Can you work these out from the model? Positions are in its coordinate system, mm. Face numbers are marked on the shaded views. A direction names the side the tool comes from. Round coordinates to 2 decimals unless told otherwise and drop trailing zeros. Loops run counter-clockwise (first coordinate to the right, second up) from the corner with the lowest first, then second, coordinate; pieces in that order, holes last. Notation, with made-up numbers: (-6.5, 9.25) -> (50.5, 9.25) arc R16 cw to (50.5, 13.25) -> close; hole circle Ø9 at (44, 52). An arc over 180 degrees is marked (long way). Write item = value, one per line.
from build123d import *

# Parameters (mm, degrees)
SKETCH2_R           = 2.1
BOSS_EXTRUDE1_DEPTH = 5
SKETCH3_R           = 5
SKETCH3_R_2         = 2.1
BOSS_EXTRUDE2_DEPTH = 5


with BuildPart() as part:
    # Sketch2 → Boss-Extrude1 (new body)
    with BuildSketch(Plane.XY):
        with BuildLine():
            ThreePointArc((-40.021658011, 2.236067977), (-48.021658011, -1.763932023), (-40.021658011, -5.763932023))
            Line((-40.021658011, -5.763932023), (-40.021658011, 2.236067977))
        make_face()
        with Locations((-43.021658011, -1.763932023)):
            Circle(SKETCH2_R, mode=Mode.SUBTRACT)
        with BuildLine():
            Line((-40.021658011, 2.236067977), (-40.021658011, -5.763932023))
            ThreePointArc((-40.021658011, -5.763932023), (-38.549522056, -4), (-38.021658011, -1.763932023))
            ThreePointArc((-38.021658011, -1.763932023), (-38.549522056, 0.472135955), (-40.021658011, 2.236067977))
        make_face()
        with BuildLine():
            ThreePointArc((-38.021658011, -1.763932023), (-38.549522056, -4), (-40.021658011, -5.763932023))
            Line((-40.021658011, -5.763932023), (3.978341989, -5.763932023))
            ThreePointArc((3.978341989, -5.763932023), (1.978341989, -1.763932023), (3.978341989, 2.236067977))
            Line((3.978341989, 2.236067977), (-40.021658011, 2.236067977))
            ThreePointArc((-40.021658011, 2.236067977), (-38.549522056, 0.472135955), (-38.021658011, -1.763932023))
        make_face()
        with BuildLine():
            Line((3.978341989, 2.236067977), (3.978341989, -5.763932023))
            ThreePointArc((3.978341989, -5.763932023), (9.214409967, -6.236067977), (11.978341989, -1.763932023))
            ThreePointArc((11.978341989, -1.763932023), (9.214409967, 2.708203932), (3.978341989, 2.236067977))
        make_face()
        with Locations((6.978341989, -1.763932023)):
            Circle(SKETCH2_R, mode=Mode.SUBTRACT)
        with BuildLine():
            ThreePointArc((3.978341989, 2.236067977), (1.978341989, -1.763932023), (3.978341989, -5.763932023))
            Line((3.978341989, -5.763932023), (3.978341989, 2.236067977))
        make_face()
    extrude(amount=BOSS_EXTRUDE1_DEPTH)

    # Sketch3 → Boss-Extrude2 (add)
    with BuildSketch(Plane.XY.offset(5)):
        with Locations((-43.021658011, -1.763932023)):
            Circle(SKETCH3_R)
        with Locations((-43.021658011, -1.763932023)):
            Circle(SKETCH3_R_2, mode=Mode.SUBTRACT)
    extrude(amount=BOSS_EXTRUDE2_DEPTH)


solid = part.part
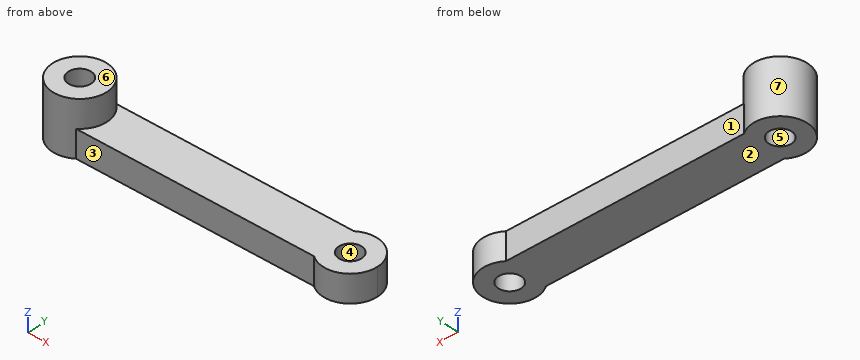
1. Suppose I cut it at D-D, the plane z = 6.25. List the corners of the cut face in (x, y) for me.
Entries:
outline = circle Ø10 at (-43.02, -1.76); hole circle Ø4.2 at (-43.02, -1.76)
2. We'd pull the mould along Y, two halves only. Please class the marked faces 4, 5, 6 and 7: released by +Y, released by -Y, zero draft, split by the parting line, or undercut.
Entries:
face_4 = undercut
face_5 = undercut
face_6 = zero draft
face_7 = split by the parting line
3. Suppose I cut it at B-B, the plane y = -2.5. List the corners of the cut face in (x, z) for me, and give its area (3 significant figures).
Entries:
outline = (-47.97, 0) -> (-44.99, 0) -> (-44.99, 10) -> (-47.97, 10) -> close; (-41.05, 0) -> (5.01, 0) -> (5.01, 5) -> (-38.08, 5) -> (-38.08, 10) -> (-41.05, 10) -> close; (8.95, 0) -> (11.92, 0) -> (11.92, 5) -> (8.95, 5) -> close
area = 290 mm²
4. Suppose I cut it at C-C, the plane x = -41.5. List the corners of the cut face in (y, z) for me, and give its area (3 significant figures).
Entries:
outline = (-6.53, 0) -> (-3.21, 0) -> (-3.21, 10) -> (-6.53, 10) -> close; (-0.32, 0) -> (3, 0) -> (3, 10) -> (-0.32, 10) -> close
area = 66.3 mm²
5. I need wall thicknesses on line 1 (Y direction, x = -43, z = 8.5); line 2 (Z direction, x = -12, y = -3.5); line 3 (Y direction, x = -12.5, z = 3.5). Which ranges of each line are inside material? Lowest first, please. Write a range as [from, to].
Entries:
line_1 = [-6.76, -3.86], [0.34, 3.24]
line_2 = [0, 5]
line_3 = [-5.76, 2.24]
6. Suppose I cut it at A-A, the plane z = 2.5. List the corners of the cut face in (x, y) for me, and give its area (3 significant figures).
Entries:
outline = (-40.02, -5.76) -> (3.98, -5.76) arc R5 ccw (long way) to (3.98, 2.24) -> (-40.02, 2.24) arc R5 ccw (long way) to start; hole circle Ø4.2 at (-43.02, -1.76); hole circle Ø4.2 at (6.98, -1.76)
area = 459 mm²
7. For the marked faces 1, 2 and 3, which set-ups out of +Z, -Z, +X, -X, +Y, -Y let a thin tool reach every point of the face, with its end or its side?
Entries:
face_1 = +Z, -Z, +Y
face_2 = -Z, +X, -X, +Y, -Y
face_3 = +Z, -Z, -Y
8. I'm going to push flat-ended pins straight in: pin 1 (1.5 mm diameter, centred on x = -18.5, z = 2.5, fed in from +Y); pin 2 (1.5 mm diameter, centred on y = 2, z = 5.5, fed in from -X); pin 3 (1.5 mm diameter, centred on x = -10, z = 2.5, fed in from -Y). Where does each tip first touch, or does it pass through?
Entries:
pin_1 = 2.24
pin_2 = -47.01
pin_3 = -5.76
